Verification items for the finished model (mm, model axes). A direction names the side the tool comes from. Give positions to 0.01 mm unless a question says otherwise; leave off trailing zeros. Write each loop counter-clockwise with the first axis right and the second up, starting at its lowest first coordinate (ties: lowest second). Pieces come first, ordered by that corner, then holes. Notation, with made-up numbers: (55.25, 56.25) - (72.25, 56.25) arc R14 cw to (72.25, 65.25) - close; hole circle Ø4 at (9, 3). An arc over 180 degrees is marked (long way). Answer as a JSON object with one key per item and string values. Group by question number.
Item 1: Sectioned sample at C-C, the plane x = -2.5. Record the boundary of the cut face in (y, z).
Item 2: Sectioned sample at D-D, the plane y = -16. Record the boundary of the cut face in (x, z).
Item 3: Scan lines: line 1 along Z through (x, y) = (-2.5, -2); line 2 along Y through (x, z) = (-3.5, -1.35); line 3 along Y through (x, z) = (3.25, -0.55). Record each from-to range of solid material in increasing order. Write a range as [from, to].
Item 4: Go/stop test with a flat-tipped pin: pin 1 (6 mm diameter, centred on x = 3, y = 2, fed in from -Z). Record where the tip stops, or that it passes through.
Item 5: Sectioned sample at B-B, the plane z = -1.25. Record the boundary of the cut face in (x, y).
Item 6: Sectioned sample at A-A, the plane y = 22.5. Record the boundary of the cut face in (x, z), and give its area (3 significant figures).
Item 7: Tool access check on faces 1 (the face through (0, 30, 1)), 2 (the face through (-0.521, 26.466, -0.986)). Record the directions out of +Z, -Z, +X, -X, +Y, -Y that give a thin tool (end or side, any length) a straight path to the whole face; none if there is none.
```python
from build123d import *

# Parameters (mm, degrees)
SKETCH1_W           = 10
SKETCH1_H           = 60
SKETCH1_R           = 4
BOSS_EXTRUDE1_DEPTH = 2
SKETCH1_3_R         = 4
BOSS_EXTRUDE2_DEPTH = 2


with BuildPart() as part:
    # Sketch1 → Boss-Extrude1 (new body)
    # profile 1 of 3: a face of its own
    with BuildSketch(Plane.XY):
        Rectangle(SKETCH1_W, SKETCH1_H)
        with Locations((0, -22.5)):
            Circle(SKETCH1_R, mode=Mode.SUBTRACT)
        with Locations((0, 22.5)):
            Circle(SKETCH1_R, mode=Mode.SUBTRACT)
    # profile 2 of 3: a face of its own
    with BuildSketch(Plane.XY):
        with Locations((0, 22.5)):
            Circle(SKETCH1_R)
    # profile 3 of 3: a face of its own
    with BuildSketch(Plane.XY):
        with Locations((0, -22.5)):
            Circle(SKETCH1_R)
    extrude(amount=BOSS_EXTRUDE1_DEPTH)

    # Sketch1_3 → Boss-Extrude2 (add)
    with BuildSketch(Plane.XY):
        with Locations((0, 22.5)):
            Circle(SKETCH1_3_R)
        with Locations((0, -22.5)):
            Circle(SKETCH1_3_R)
    extrude(amount=-BOSS_EXTRUDE2_DEPTH)


solid = part.part
```
Geometry check:
{
 "1": {"outline": "(-30, 0) - (-25.62, 0) - (-25.62, -2) - (-19.38, -2) - (-19.38, 0) - (19.38, 0) - (19.38, -2) - (25.62, -2) - (25.62, 0) - (30, 0) - (30, 2) - (-30, 2) - close"},
 "2": {"outline": "(-5, 0) - (5, 0) - (5, 2) - (-5, 2) - close"},
 "3": {"line 1": "[0, 2]", "line 2": "[-24.44, -20.56], [20.56, 24.44]", "line 3": "[-24.83, -20.17], [20.17, 24.83]"},
 "4": {"pin 1": "z = 0"},
 "5": {"outline": "circle Ø8 at (0, -22.5); circle Ø8 at (0, 22.5)"},
 "6": {"outline": "(-5, 0) - (-4, 0) - (-4, -2) - (4, -2) - (4, 0) - (5, 0) - (5, 2) - (-5, 2) - close", "area": "36.0 mm^2"},
 "7": {"face 1": "+Z, -Z, +X, -X, +Y", "face 2": "-Z"}
}
